Work out the finished part from the listing and answer in its coordinate system (mm). Face numbers are marked on the shaded views. Coordinates: 2 decimals unless noted, no trailing zeros. Loops run counter-clockwise (first coordinate to the right, second up) from the corner with the lowest first, then second, coordinate; pieces in that order, holes last.
```python
from build123d import *

# Parameters (mm, degrees)
F0_W     = 70
F0_H     = 28
F1_DEPTH = 200
F2_R     = 14
F3_DEPTH = 28.001
F4_R     = 5
F5_R     = 1


with BuildPart() as f1:
    # F0 (on Front) → F1 (new body)
    with BuildSketch(Plane.XZ):
        Rectangle(F0_W, F0_H)
    extrude(amount=F1_DEPTH)

    # F2 (on face) → F3 (cut, through all)
    with BuildSketch(Plane.XY.offset(14)):
        Circle(F2_R)
    extrude(amount=-F3_DEPTH, mode=Mode.SUBTRACT)

    # F4
    f4_edges = [f1.edges().sort_by_distance(p)[0] for p in [
        (-35, -100, 14),
        (35, -100, 14),
        (35, -100, -14),
        (-35, -100, -14),
        (0, -200, 14),
        (0, -200, -14),
        (35, -200, 0),
        (-35, -200, 0),
    ]]
    fillet(f4_edges, radius=F4_R)

    # F5
    f5_edges = [f1.edges().sort_by_distance(p)[0] for p in [
        (0, -14, -14),
        (0, -14, 14),
    ]]
    fillet(f5_edges, radius=F5_R)


solid = f1.part
```
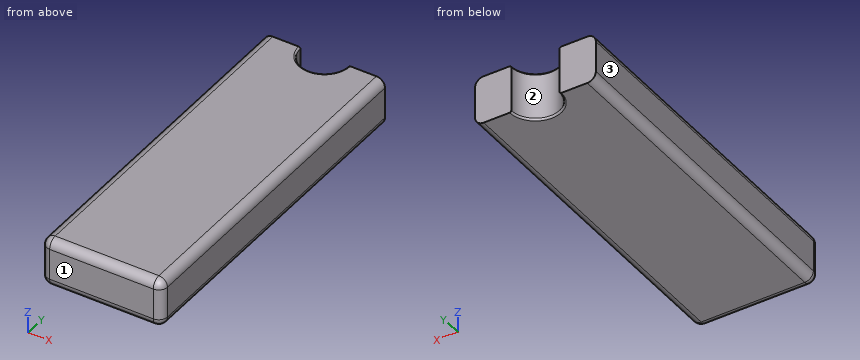
1. Straight lines are drawn through the part: probe 1 along X at (y, z) = (-151, 9.5); probe 2 along Y at (x, z) = (0, 9.25); probe 3 along X at (y, z) = (-165, -12.25). For each, find the intervals that lie inside material, in ascending order.
2. Determine the mould class of the marked faces 1, 2 and 3 for opening direction X: released by +X, released by -X, zero draft, split by the parting line, or undercut.
3. A cutting plane is placed at A-A, the plane z = 3. Give the vertices of the cut face in (x, y).
4. Each of these flat-tipped pins is pushed along its axis until it touches: P1, Ø5, axis at x = -8.5, z = -6.5, coming from the +Y side; P2, Ø1, axis at y = -167, z = -11, coming from the +X side. Where does it stop, or does it pass through?
5. A cutting plane is placed at B-B, the plane x = 0. Give the vertices of the cut face in (y, z).
Answers below:
1. probe 1: x = -34.97 to 34.97
1. probe 2: y = -199.99 to -14
1. probe 3: x = -33.8 to 33.8
2. face 1: zero draft
2. face 2: undercut
2. face 3: released by -X
3. outline: (-35, -195) arc R5 ccw to (-30, -200) - (30, -200) arc R5 ccw to (35, -195) - (35, 0) - (14, 0) arc R14 cw to (-14, 0) - (-35, 0) - close
4. P1: stops at y = -8.66
4. P2: stops at x = 34.77
5. outline: (-200, -9) arc R5 ccw to (-195, -14) - (-15, -14) arc R1 ccw to (-14, -13) - (-14, 13) arc R1 ccw to (-15, 14) - (-195, 14) arc R5 ccw to (-200, 9) - close
